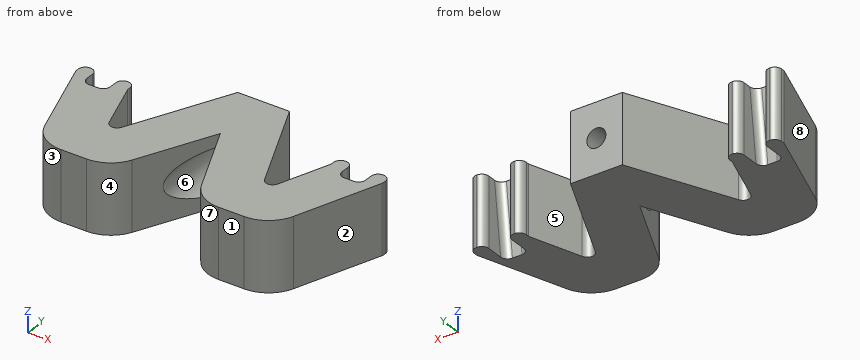
from build123d import *

# Parameters (mm, degrees)
SKETCH1_R           = 4
BOSS_EXTRUDE1_DEPTH = 20
FILLET1_R           = 10
SKETCH2_W           = 6.75
SKETCH2_H           = 6.75
CUT_EXTRUDE1_DEPTH  = 122.829645635
SKETCH3_W           = 4.125
SKETCH3_H           = 20
BOSS_EXTRUDE2_DEPTH = 3
FILLET2_R           = 2
BOSS_EXTRUDE3_DEPTH = 20
SKETCH6_W           = 140
SKETCH6_H           = 64.976574758
CUT_EXTRUDE3_DEPTH  = 133.326301241
SKETCH7_R           = 6.5
CUT_EXTRUDE4_DEPTH  = 35.523425242
FILLET5_R           = 2
FILLET6_R           = 10
SKETCH8_R           = 2.75
CUT_EXTRUDE5_DEPTH  = 61.35034168


with BuildPart() as part:
    # Sketch1 → Boss-Extrude1 (new body)
    with BuildSketch(Plane.XY):
        with BuildLine():
            Line((-70, 0), (70, 0))
            Line((70, 0), (70, 12))
            ThreePointArc((70, 12), (66.338834765, 20.838834765), (57.5, 24.5))
            Line((57.5, 24.5), (25, 24.5))
            Line((25, 24.5), (25, 39.5))
            Line((25, 39.5), (44.5, 96.5))
            Line((44.5, 96.5), (29.5, 96.5))
            Line((29.5, 96.5), (0, 10.269230769))
            Line((0, 10.269230769), (-29.5, 96.5))
            Line((-29.5, 96.5), (-44.5, 96.5))
            Line((-44.5, 96.5), (-25, 39.5))
            Line((-25, 39.5), (-25, 24.5))
            Line((-25, 24.5), (-57.5, 24.5))
            ThreePointArc((-57.5, 24.5), (-66.338834765, 20.838834765), (-70, 12))
            Line((-70, 12), (-70, 0))
        make_face()
        with Locations((-57.5, 12)):
            Circle(SKETCH1_R, mode=Mode.SUBTRACT)
        with Locations(Location((57.5, 12, 0), (0, 0, 180))):
            Circle(SKETCH1_R, mode=Mode.SUBTRACT)
    extrude(amount=BOSS_EXTRUDE1_DEPTH)

    # Fillet1
    fillet1_edges = [part.edges().sort_by_distance(p)[0] for p in [
        (25, 39.5, 10),
        (25, 24.5, 10),
        (-25, 24.5, 10),
        (-25, 39.5, 10),
        (0, 10.269230769, 10),
    ]]
    fillet(fillet1_edges, radius=FILLET1_R)

    # Sketch2 → Cut-Extrude1 (cut, through all, along a direction that is not the sketch's normal)
    with BuildSketch(Plane.XY.offset(20)):
        with Locations((37, 96.5)):
            Rectangle(SKETCH2_W, SKETCH2_H)
        with Locations((-37, 96.5)):
            Rectangle(SKETCH2_W, SKETCH2_H)
    extrude(amount=-CUT_EXTRUDE1_DEPTH, dir=(0, 0.12403473458920856, 0.9922778767136676), mode=Mode.SUBTRACT)

    # Sketch3 → Boss-Extrude2 (add)
    with BuildSketch(Plane(origin=(0, 96.5, 0), x_dir=(1, 0, 0), z_dir=(0, 1, 0))):
        with Locations((42.4375, -10)):
            Rectangle(SKETCH3_W, SKETCH3_H)
        with Locations((31.5625, -10)):
            Rectangle(SKETCH3_W, SKETCH3_H)
        with Locations((-31.5625, -10)):
            Rectangle(SKETCH3_W, SKETCH3_H)
        with Locations((-42.4375, -10)):
            Rectangle(SKETCH3_W, SKETCH3_H)
    extrude(amount=BOSS_EXTRUDE2_DEPTH)

    # Fillet2
    fillet2_edges = [part.edges().sort_by_distance(p)[0] for p in [
        (40.375, 91.875, 10),
        (33.625, 91.875, 10),
        (44.5, 99.5, 10),
        (40.375, 99.5, 10),
        (29.5, 99.5, 10),
        (33.625, 99.5, 10),
        (-29.5, 99.5, 10),
        (-33.625, 99.5, 10),
        (-44.5, 99.5, 10),
        (-40.375, 99.5, 10),
        (44.5, 96.5, 10),
        (-33.625, 91.875, 10),
        (-40.375, 91.875, 10),
    ]]
    fillet(fillet2_edges, radius=FILLET2_R)

    # Sketch4 → Boss-Extrude3 (add)
    with BuildSketch(Plane.XY.offset(20)):
        Polygon((-22.82093347, 76.976574758), (-7.5, 110.5), (7.5, 110.5), (22.82093347, 76.976574758), (16.14070638, 57.44975711), (0, 92.766910908), (-16.14070638, 57.44975711), align=None)
    extrude(amount=-BOSS_EXTRUDE3_DEPTH)

    # Sketch6 → Cut-Extrude3 (cut, through all)
    with BuildSketch(Plane.XY.offset(20)):
        with Locations((0, 32.488287379)):
            Rectangle(SKETCH6_W, SKETCH6_H)
    extrude(amount=-CUT_EXTRUDE3_DEPTH, mode=Mode.SUBTRACT)

    # Sketch7 → Cut-Extrude4 (cut)
    with BuildSketch(Plane.XZ.offset(-64.976574758)):
        with Locations(Location((0, 10, 0), (0, 0, 90))):
            Circle(SKETCH7_R)
    extrude(amount=-CUT_EXTRUDE4_DEPTH, mode=Mode.SUBTRACT)

    # Fillet5
    fillet5_edges = [part.edges().sort_by_distance(p)[0] for p in [
        (22.82093347, 76.976574758, 10),
        (-22.82093347, 76.976574758, 10),
    ]]
    fillet(fillet5_edges, radius=FILLET5_R)

    # Fillet6
    fillet6_edges = [part.edges().sort_by_distance(p)[0] for p in [
        (12.700787231, 64.976574758, 10),
        (-33.715670312, 64.976574758, 10),
        (33.715670312, 64.976574758, 10),
        (-12.700787231, 64.976574758, 10),
    ]]
    fillet(fillet6_edges, radius=FILLET6_R)

    # Sketch8 → Cut-Extrude5 (cut, through all)
    with BuildSketch(Plane.XZ.offset(-100.5)):
        with Locations(Location((0, 10, 0), (0, 0, 270))):
            Circle(SKETCH8_R)
    extrude(amount=-CUT_EXTRUDE5_DEPTH, mode=Mode.SUBTRACT)


solid = part.part
The listing builds one solid part. Answer for the finished solid, in the listing's coordinates (mm). Face numbers are marked on the shaded views. A direction names the side the tool comes from. Coordinates: 2 decimals unless noted, no trailing zeros. Write each loop counter-clockwise with the first axis right and the second up, starting at its lowest first coordinate (ties: lowest second). Pieces come first, ordered by that corner, then holes. Notation, with made-up numbers: M -18.75,77 L 2.25,77 A20 cw 2.25,109 Z; hole C 25.5,66.25 d5. An arc over 180 degrees is marked long. Write each question's results on one line, items separated by ' | '.
Item 1: The part is cut by section C-C on x = -32.5. Determine the outline of the cut face in (y, z).
Answer below:
outline: M 66.93,0 L 99.3,0 L 99.3,20 L 66.93,20 Z
Item 2: The part is cut by section B-B on x = -5. Determine the outline of the cut face in (y, z), and give its area (3 significant figures).
Answer below:
outline: M 81.83,0 L 110.5,0 L 110.5,20 L 81.83,20 L 81.83,14.15 L 100.5,14.15 L 100.5,5.85 L 81.83,5.85 Z | area: 418 mm2
Item 3: The part is cut by section A-A on y = 85.5. Determine the outline of the cut face in (x, z), and give its area (3 significant figures).
Answer below:
outline: M -40.74,0 L -25.74,0 L -25.74,20 L -40.74,20 Z; M -18.93,0 L -3.32,0 L -3.32,4.41 A6.5 cw -3.32,15.59 L -3.32,20 L -18.93,20 Z; M 3.32,0 L 18.93,0 L 18.93,20 L 3.32,20 L 3.32,15.59 A6.5 cw 3.32,4.41 Z; M 25.74,0 L 40.74,0 L 40.74,20 L 25.74,20 Z | area: 1,170 mm2
Item 4: Given P1, Ø1.5, axis at x = 19.5, z = 13, coming from the +Y side; P2, Ø6.5, axis at x = 1, z = 10, coming from the -Y side; P3, Ø5, axis at x = -34.5, z = 18, coming from the +Y side, each flat-ended and moving along its own axis, determine where each tip first touches the part or whether it passes through.
Answer below:
P1: y = 85.88 | P2: y = 100.5 | P3: y = 99.46
Item 5: The part is cut by section D-D on x = 18. Determine the outline of the cut face in (y, z), and give its area (3 significant figures).
Answer below:
outline: M 65.04,0 L 87.53,0 L 87.53,20 L 65.04,20 Z | area: 450 mm2
Item 6: Consider probe 1 along X at (y, z) = (84.5, 10); probe 2 along X at (y, z) = (96, 12) (3 decimals); probe 3 along X at (y, z) = (85.5, 10). Determine where each line is inside the solid, lowest interval first. Write a range as [from, to].
Answer below:
probe 1: [-40.39, -25.39], [-19.38, -6.5], [6.5, 19.38], [25.39, 40.39] | probe 2: [-44.329, -40.375], [-33.625, -29.329], [-14.127, -6.185], [6.185, 14.127], [29.329, 33.625], [40.375, 44.329] | probe 3: [-40.74, -25.74], [-18.93, -6.5], [6.5, 18.93], [25.74, 40.74]
Item 7: For a pull along X with two mould halves and no side action, classify the marked faces 1, 2, 3 and 4 as released by +X, released by -X, zero draft, split by the parting line, or undercut.
Answer below:
face 1: zero draft | face 2: released by +X | face 3: released by -X | face 4: undercut
Item 8: Which of the six approach directions +Z, -Z, +X, -X, +Y, -Y give full straight-line access (tool end or side, diameter ignored) to the marked faces 5, 6, 7 and 8?
Answer below:
face 5: +Z, -Z, +Y | face 6: -Y | face 7: +Z, -Z, -Y | face 8: +Z, -Z, -X, -Y
